Geometry: final body of the model. Coordinates: model frame, mm. A direction names the side the tool comes from. Coordinates: 2 decimals unless noted, no trailing zeros. Loops run counter-clockwise (first coordinate to the right, second up) from the corner with the lowest first, then second, coordinate; pieces in that order, holes last. Notation, with made-up numbers: (-1, -6.75) - (57, -6.75) arc R8 cw to (57, 7.25) - close; hole circle Ø4 at (76, 88.25). An arc over 180 degrees is marked (long way). Answer in a Markdown table with one row per item.
from build123d import *

# Parameters (mm, degrees)
SKETCH1_R                = 27.5
SKETCH1_R_2              = 15
BOSS_EXTRUDE1_DEPTH      = 10
SKETCH2_R                = 55.75
SKETCH2_R_2              = 27.5
BOSS_EXTRUDE2_DEPTH      = 2.5
BOSS_EXTRUDE2_DEPTH_BACK = 2.5


with BuildPart() as part:
    # Sketch1 → Boss-Extrude1 (new body)
    with BuildSketch(Plane.XY):
        Circle(SKETCH1_R)
        Circle(SKETCH1_R_2, mode=Mode.SUBTRACT)
    extrude(amount=BOSS_EXTRUDE1_DEPTH)

    # Sketch2 → Boss-Extrude2 (add, two sides)
    with BuildSketch(Plane.XY.offset(5)) as boss_extrude2_sk:
        Circle(SKETCH2_R)
        Circle(SKETCH2_R_2, mode=Mode.SUBTRACT)
    extrude(amount=BOSS_EXTRUDE2_DEPTH)
    extrude(boss_extrude2_sk.sketch, amount=-BOSS_EXTRUDE2_DEPTH_BACK)


solid = part.part
(1) Cut plane C-C on z = 5. Output: boundary loops of the cut face in (x, y), then the cut area to 3 significant figures.
Verdict:
| item | result |
|---|---|
| outline | circle Ø111.5 at (0, 0); hole circle Ø30 at (0, 0) |
| area | 9,060 mm² |
(2) Ray query, probe 1 along Y at (x, z) = (0, 3.75); probe 2 along Z at (x, y) = (29.5, 46); probe 3 along X at (y, z) = (25.5, 4.75). Return the intervals inside material, ascending.
Verdict:
| item | result |
|---|---|
| probe 1 | y = -55.75 to -15, 15 to 55.75 |
| probe 2 | z = 2.5 to 7.5 |
| probe 3 | x = -49.58 to 49.58 |
(3) First-contact query: pin 1 Ø5 at (y, z) = (-15.5, 6) entering from +X; pin 2 Ø12 at (x, y) = (-27.5, -19) entering from +Z; pin 3 Ø12 at (x, y) = (-43, 17.5) entering from -Z; pin 4 Ø4 at (x, z) = (-31, 5) entering from -Y. Flat tips, straight axial feed; report the tip coordinate or a pass-through.
Verdict:
| item | result |
|---|---|
| pin 1 | stops at x = 54.21 |
| pin 2 | stops at z = 10 |
| pin 3 | stops at z = 2.5 |
| pin 4 | stops at y = -47.61 |
(4) Cut plane A-A on x = 0. Output: boundary loops of the cut face in (y, z), then the cut area to 4 significant figures.
Verdict:
| item | result |
|---|---|
| outline | (-55.75, 2.5) - (-27.5, 2.5) - (-27.5, 0) - (-15, 0) - (-15, 10) - (-27.5, 10) - (-27.5, 7.5) - (-55.75, 7.5) - close; (15, 0) - (27.5, 0) - (27.5, 2.5) - (55.75, 2.5) - (55.75, 7.5) - (27.5, 7.5) - (27.5, 10) - (15, 10) - close |
| area | 532.5 mm² |
(5) Access query for faces 1 (the face through (12, 26, 2.5)), 2 (the face through (-7.258, 55.276, 5.035)). Directions: +Z, -Z, +X, -X, +Y, -Y. A direction counts if a zero-diameter tool reaches every point of the face in a straight line with its end or side. Return the directions, or none.
Verdict:
| item | result |
|---|---|
| face 1 | -Z |
| face 2 | +Z, -Z |
(6) Pull-direction query (Y, two-part tool) for faces 3 (the face through (12, 26, 7.5)), 4 (the face through (-5.961, -26.846, 8.732)), 5 (the face through (-14.985, 0.66, 4.93)); classes: pulls with the +Y half, pulls with the -Y half, needs draft (parallel to the pull), parting line crosses it, or undercut.
Verdict:
| item | result |
|---|---|
| face 3 | needs draft |
| face 4 | parting line crosses it |
| face 5 | undercut |
(7) Cut plane D-D on x = 19.5. Output: boundary loops of the cut face in (y, z), then the cut area to 3 significant figures.
Verdict:
| item | result |
|---|---|
| outline | (-52.23, 2.5) - (-19.39, 2.5) - (-19.39, 0) - (19.39, 0) - (19.39, 2.5) - (52.23, 2.5) - (52.23, 7.5) - (19.39, 7.5) - (19.39, 10) - (-19.39, 10) - (-19.39, 7.5) - (-52.23, 7.5) - close |
| area | 716 mm² |
